Build history of the part. All positions in model axes, mm. A direction names the side the tool comes from. Coordinates: 2 decimals unless noted, no trailing zeros. Order: outer loops, then holes, each group sorted by start corner. A loop starts at its lowest first (then second) coordinate and runs counter-clockwise, first axis right, second up. Notation, with made-up numbers: (44.5, -24) - (83.5, -24) arc R19 ccw to (83.5, 1) - close; hole circle Ø11 at (-37, -38.75). An arc over 180 degrees is marked (long way). Return JSON: item names as keys, results as strings.
Autodesk Inventor part; units mm, degrees
ref_plane "YZ Plane" through (0, 0, 0) normal (1, 0, 0) x (0, 1, 0)
ref_plane "XZ Plane" through (0, 0, 0) normal (0, 1, 0) x (-1, 0, 0)
ref_plane "XY Plane" through (0, 0, 0) normal (0, 0, 1) x (1, 0, 0)
sketch "Sketch1" plane through (0, 0, 0) normal (0, 1, 0) x (-1, 0, 0)
  line L0 (0, 0) -> (76.2, 0)
  line L1 (76.2, 0) -> (76.2, -30.48)
  line L2 (76.2, -30.48) -> (0, -30.48)
  line L3 (0, -30.48) -> (0, 0)
  dimension "d0" = 76.2
  dimension "d1" = 30.48
extrude "Extrusion1" add sketch "Sketch1" along normal blind 8.89
fillet "Fillet1" radius 3.175 8 edges at (0, 4.445, 0) (0, 4.445, -30.48) (0, 0, -15.24) (-38.1, 0, 0) (-76.2, 4.445, 0) (-76.2, 0, -15.24) (-76.2, 4.445, -30.48) (-38.1, 0, -30.48)
shell "Shell1" thickness 2.54 removed faces 1 at (-26.4583, 8.89, -20.32)
sketch "Sketch2" plane through (0, 8.89, 0) normal (0, 1, 0) x (1, 0, 0)
  arc A0 (-76.2, 3.175) -> (-73.025, 0) centre (-73.025, 3.175) ccw
  line L0 (-76.2, 27.305) -> (-76.2, 3.175)
  arc A1 (-73.025, 30.48) -> (-76.2, 27.305) centre (-73.025, 27.305) ccw
  line L1 (-3.175, 30.48) -> (-73.025, 30.48)
  line L2 (-73.025, 0) -> (-3.175, 0)
  arc A2 (-3.175, 0) -> (0, 3.175) centre (-3.175, 3.175) ccw
  line L3 (0, 3.175) -> (0, 27.305)
  arc A3 (0, 27.305) -> (-3.175, 30.48) centre (-3.175, 27.305) ccw
  arc A4 (-73.025, 29.21) -> (-74.93, 27.305) centre (-73.025, 27.305) ccw
  line L4 (-74.93, 27.305) -> (-74.93, 3.175)
  arc A5 (-74.93, 3.175) -> (-73.025, 1.27) centre (-73.025, 3.175) ccw
  line L5 (-73.025, 1.27) -> (-3.175, 1.27)
  arc A6 (-3.175, 1.27) -> (-1.27, 3.175) centre (-3.175, 3.175) ccw
  line L6 (-1.27, 3.175) -> (-1.27, 27.305)
  arc A7 (-1.27, 27.305) -> (-3.175, 29.21) centre (-3.175, 27.305) ccw
  line L7 (-3.175, 29.21) -> (-73.025, 29.21)
  point P0 (0, 0)
  dimension "d6" = 1.27
extrude "Extrusion2" cut sketch "Sketch2" against normal blind 1.27
sketch "Sketch3" plane through (0, 3.175, -3.175) normal (1, 0, 0) x (0, 0, -1)
  line L0 (0, 5.715) -> (24.13, 5.715)
  line L1 (12.065, 5.715) -> (12.065, 0.3712)
  line L2 (13.6525, 5.715) -> (13.6525, 1.5875)
  line L3 (10.4775, 5.715) -> (10.4775, 1.5875)
  line L4 (12.065, 0) -> (12.065, 0)
  arc A0 (10.4775, 1.5875) -> (12.065, 0) centre (12.065, 1.5875) ccw
  arc A1 (12.065, 0) -> (13.6525, 1.5875) centre (12.065, 1.5875) ccw
  line L5 (10.4775, 5.715) -> (13.6525, 5.715)
  point P0 (-3.175, -3.175)
  dimension "d9" = 1.5875
  dimension "d10" = 1.5875
  dimension "d11" = 5.715
  dimension "d12" = 1.5875
extrude "Extrusion3" cut sketch "Sketch3" against normal blind 2.54
properties part number "box_bottom"
1. Probe L1, parallel to Z at x = -66.5, y = 3.75; L2, parallel to X at y = 8, z = -19; L3, parallel to Z at x = -5, y = 7.75. List the from-to ranges inside material, lowest first.
Check values:
{"L1": "-30.48 to -27.94, -2.54 to 0", "L2": "-74.93 to -73.66, -2.54 to -1.27", "L3": "-29.21 to -27.94, -2.54 to -1.27"}
2. Drop flat-ended pins along their axis: pin 1 (15 mm diameter, centred on x = -23, z = -18.5, fed in from +Y); pin 2 (0.6 mm diameter, centred on x = -47.5, y = 8.5, fed in from +Z); pin 3 (0.6 mm diameter, centred on x = -42, y = 8, fed in from -Z). Give the stop position or say it passes through.
Check values:
{"pin 1": "y = 2.54", "pin 2": "z = -1.27", "pin 3": "z = -29.21"}
3. Tool access for faces 1 (the flat face through (-39, 8, -1.27)), 2 (the flat face through (-2.54, 6, -9)), 3 (the flat face through (-1.27, 8, -22)): list every direction of +Z, -Z, +X, -X, +Y, -Y with a clear straight run to the whole face (end or side of a thin tool).
Check values:
{"face 1": "+Z, +X, -X, +Y", "face 2": "+Y", "face 3": "+Z, -Z, +X, +Y"}
4. Cut at B-B on x = -6.5. Give the cut face in (y, z) (3 decimals), plus the area to 3 significant figures.
Check values:
{"outline": "(0, -27.305) arc R3.175 ccw to (3.175, -30.48) - (7.62, -30.48) - (7.62, -29.21) - (8.89, -29.21) - (8.89, -27.94) - (3.175, -27.94) arc R0.635 cw to (2.54, -27.305) - (2.54, -3.175) arc R0.635 cw to (3.175, -2.54) - (8.89, -2.54) - (8.89, -1.27) - (7.62, -1.27) - (7.62, 0) - (3.175, 0) arc R3.175 ccw to (0, -3.175) - close", "area": "102 mm²"}
5. Mould opens along X. For faces 4 (the flat face through (-38, 0, -15)), 5 (the flat face through (-2.54, 6, -23)), 6 (the cylindrical face through (-0.95, 5.43, -0.91)) say: pulls with the +X half, pulls with the -X half, needs draft (parallel to the pull), parting line crosses it, or undercut.
Check values:
{"face 4": "needs draft", "face 5": "undercut", "face 6": "pulls with the +X half"}
6. Cut at C-C on z = -20. Give the cut face in (x, y) (3 decimals).
Check values:
{"outline": "(-76.2, 3.175) arc R3.175 ccw to (-73.025, 0) - (-3.175, 0) arc R3.175 ccw to (0, 3.175) - (0, 7.62) - (-1.27, 7.62) - (-1.27, 8.89) - (-2.54, 8.89) - (-2.54, 3.175) arc R0.635 cw to (-3.175, 2.54) - (-73.025, 2.54) arc R0.635 cw to (-73.66, 3.175) - (-73.66, 8.89) - (-74.93, 8.89) - (-74.93, 7.62) - (-76.2, 7.62) - close"}
7. Cut at D-D on z = -14.5. Give the cut face in (x, y) (3 decimals), plus the area to 3 significant figures.
Check values:
{"outline": "(-76.2, 3.175) arc R3.175 ccw to (-73.025, 0) - (-3.175, 0) arc R3.175 ccw to (0, 3.175) - (0, 3.358) - (-2.54, 3.358) - (-2.54, 3.175) arc R0.635 cw to (-3.175, 2.54) - (-73.025, 2.54) arc R0.635 cw to (-73.66, 3.175) - (-73.66, 8.89) - (-74.93, 8.89) - (-74.93, 7.62) - (-76.2, 7.62) - close", "area": "206 mm²"}
